Can you work these out from the model? Positions are in its coordinate system, mm. Give positions to 0.01 mm unless a question says otherwise; leave off trailing zeros. Order: outer loops, then holes, each group sorted by start corner. A loop starts at its lowest first (then second) coordinate and runs counter-clockwise, first axis right, second up. Notation, with made-up numbers: (-14.5, -35) - (-6.5, -35) arc R33 cw to (-6.5, 1) - close; hole circle Ø10 at (74.25, 40.5). An arc over 180 degrees is marked (long way). One line per question, with ' | ' between items.
Autodesk Fusion 360 part; units mm, degrees
sketch "Sketch1" plane through (0, 0, 0) normal (1, 0, 0) x (0, 1, 0)
  circle A0 centre (0, 0) radius 15
  line L0 (6.3897, -13.8986) -> (5.9544, -13.7676)
  line L1 (0, 15) -> (0, 23)
  line L2 (0, 15) -> (-3, 15)
  line L3 (0, 15) -> (3, 15)
  line L4 (0, 23) -> (3, 15)
  line L5 (0, 23) -> (-3, 15)
  line L6 (-3, 15) -> (-3.1925, 14.4866)
  line L7 (3, 15) -> (3.1794, 14.5216)
  circle A1 centre (0, 0) radius 15
  circle A2 centre (0, 0) radius 15
  line L8 (-23, 0) -> (-15, -3)
  line L9 (-23, 0) -> (-15, 3)
  line L10 (-15, 3) -> (-14.5216, 3.1794)
  line L11 (-15, -3) -> (-14.4866, -3.1925)
  circle A3 centre (0, 0) radius 15
  line L12 (0, -23) -> (3, -15)
  line L13 (0, -23) -> (-3, -15)
  line L14 (-3, -15) -> (-3.1794, -14.5216)
  line L15 (3, -15) -> (3.1925, -14.4866)
  circle A4 centre (0, 0) radius 15
  line L16 (23, 0) -> (15, 3)
  line L17 (23, 0) -> (15, -3)
  line L18 (15, -3) -> (14.5216, -3.1794)
  line L19 (15, 3) -> (14.4866, 3.1925)
  circle A5 centre (0, 0) radius 15
  dimension "d1" = 30
  dimension "d16" = 8
  dimension "d17" = 3
  dimension "d18" = 3
  dimension "d31" = 360
extrude "Extrude9" add sketch "Sketch1" along normal blind 60
sketch "Sketch8" plane through (60, 0, 0) normal (1, 0, 0) x (0, 1, 0)
  line L0 (23, 0) -> (14.6712, 3.1233)
  arc A0 (14.6712, 3.1233) -> (3.1233, 14.6712) centre (0, 0) ccw
  line L1 (3.1233, 14.6712) -> (0, 23)
  line L2 (0, 23) -> (-3.1233, 14.6712)
  arc A1 (-3.1233, 14.6712) -> (-14.6712, 3.1233) centre (0, 0) ccw
  line L3 (-14.6712, 3.1233) -> (-23, 0)
  line L4 (-23, 0) -> (-14.6712, -3.1233)
  arc A2 (-14.6712, -3.1233) -> (-3.1233, -14.6712) centre (0, 0) ccw
  line L5 (-3.1233, -14.6712) -> (0, -23)
  line L6 (0, -23) -> (3.1233, -14.6712)
  arc A3 (3.1233, -14.6712) -> (14.6712, -3.1233) centre (0, 0) ccw
  line L7 (14.6712, -3.1233) -> (23, 0)
  circle A4 centre (0, 0) radius 2.4
  dimension "d34" = 4.8
extrude "Extrude10" cut sketch "Sketch8" against normal blind 85 contours A4
sketch "Sketch9" plane through (60, 0, 0) normal (1, 0, 0) x (0, 1, 0)
  circle A0 centre (0, 0) radius 2.4
  line L0 (23, 0) -> (14.6712, 3.1233)
  arc A1 (14.6712, 3.1233) -> (3.1233, 14.6712) centre (0, 0) ccw
  line L1 (3.1233, 14.6712) -> (0, 23)
  line L2 (0, 23) -> (-3.1233, 14.6712)
  arc A2 (-3.1233, 14.6712) -> (-14.6712, 3.1233) centre (0, 0) ccw
  line L3 (-14.6712, 3.1233) -> (-23, 0)
  line L4 (-23, 0) -> (-14.6712, -3.1233)
  arc A3 (-14.6712, -3.1233) -> (-3.1233, -14.6712) centre (0, 0) ccw
  line L5 (-3.1233, -14.6712) -> (0, -23)
  line L6 (0, -23) -> (3.1233, -14.6712)
  arc A4 (3.1233, -14.6712) -> (14.6712, -3.1233) centre (0, 0) ccw
  line L7 (14.6712, -3.1233) -> (23, 0)
  circle A5 centre (0, 0) radius 23
  circle A6 centre (0, 0) radius 15
extrude "Extrude11" cut sketch "Sketch9" against normal blind 75 contours L0 L7 A6 | L1 L2 A6 | L5 L6 A6 | L3 L4 A6
sketch "Sketch10" plane through (0, 0, 0) normal (1, 0, 0) x (0, 1, 0)
  circle A0 centre (0, 0) radius 23
  circle A1 centre (0, 0) radius 15.0333
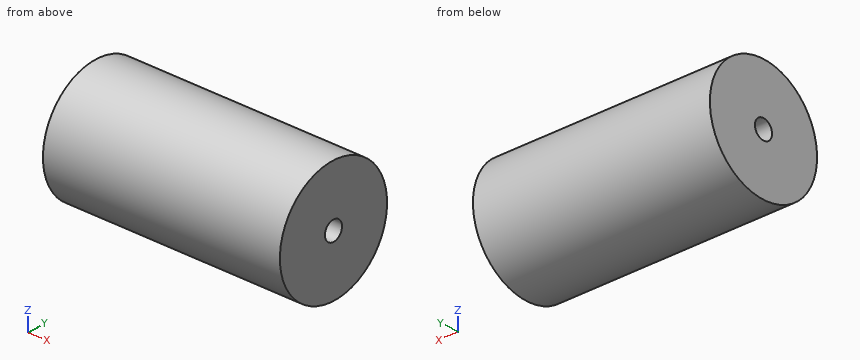
(1) Imagine slicing it at C-C (y = 9). List the corners of the cut face in (x, z) for me.
Answer below:
outline: (0, -12) - (60, -12) - (60, 12) - (0, 12) - close
(2) Imagine slicing it at D-D (x = 44). List the corners of the cut face in (y, z) for me, and give its area (3 significant figures).
Answer below:
outline: circle Ø30 at (0, 0); hole circle Ø4.8 at (0, 0) | area: 689 mm^2
(3) Imagine slicing it at A-A (y = 0). List the corners of the cut face in (x, z) for me.
Answer below:
outline: (0, -15) - (60, -15) - (60, -2.4) - (0, -2.4) - close; (0, 2.4) - (60, 2.4) - (60, 15) - (0, 15) - close
(4) If I drill on line 1 (Z direction, x = 15, y = 0); line 2 (Z direction, x = 9, y = -2); line 3 (Y direction, x = 53, z = 10), over which ranges is the centre line in solid material (lowest first)?
Answer below:
line 1: -15 to -2.4, 2.4 to 15 | line 2: -14.87 to -1.33, 1.33 to 14.87 | line 3: -11.18 to 11.18
(5) Will these pins go through, and if not, where does the flat tip stop? pin 1 (1 mm diameter, centred on x = 51.5, z = 2.5, fed in from -Y); pin 2 (5 mm diameter, centred on x = 8, y = 3, fed in from -Z); pin 3 (2 mm diameter, centred on x = 52, z = -9, fed in from -Y).
Answer below:
pin 1: y = -14.87 | pin 2: z = -14.99 | pin 3: y = -12.69
